Design review of the part built by this model. Coordinates are the model's own, in mm. A direction names the side the tool comes from. Give positions to 0.01 mm unless a question says otherwise; leave off trailing zeros. Write each loop counter-clockwise with the first axis right and the second up, starting at its lowest first coordinate (ties: lowest second). Pieces come first, ordered by that corner, then holes. Notation, with made-up numbers: (8, -36.5) - (50, -36.5) arc R11 ccw to (50, -30.5) - close; hole circle Ø3 at (-30.5, -18). An arc over 180 degrees is marked (long way). Write each question's results on one line, items separated by ' | '. Start each with the question number.
from build123d import *

# Parameters (mm, degrees)
SKETCH_1_W          = 10
SKETCH_1_H          = 10
SKETCH_1_W_2        = 8
SKETCH_1_H_2        = 8
EXTRUDE_1_DEPTH     = 225
SKETCH_2_R          = 2.1
CUT_EXTRUDE_1_DEPTH = 226.277606521
SKETCH_3_R          = 2.1
CUT_EXTRUDE_2_DEPTH = 226.277606521


with BuildPart() as part:
    # ｽｹｯﾁ1 → 押し出し-薄板1 (new body)
    with BuildSketch(Plane(origin=(0, 0, 0), x_dir=(0, 0, -1), z_dir=(1, 0, 0))):
        Rectangle(SKETCH_1_W, SKETCH_1_H)
        Rectangle(SKETCH_1_W_2, SKETCH_1_H_2, mode=Mode.SUBTRACT)
    extrude(amount=EXTRUDE_1_DEPTH)

    # ｽｹｯﾁ2 → ｶｯﾄ - 押し出し1 (cut, through all)
    with BuildSketch(Plane(origin=(0, 5, 0), x_dir=(1, 0, 0), z_dir=(0, 1, 0))):
        with Locations(Location((195, 0, 0), (0, 0, 270))):
            Circle(SKETCH_2_R)
        with Locations(Location((220, 0, 0), (0, 0, 270))):
            Circle(SKETCH_2_R)
        with Locations(Location((5, 0, 0), (0, 0, 270))):
            Circle(SKETCH_2_R)
        with Locations(Location((30, 0, 0), (0, 0, 270))):
            Circle(SKETCH_2_R)
    extrude(amount=-CUT_EXTRUDE_1_DEPTH, mode=Mode.SUBTRACT)

    # ｽｹｯﾁ3 → ｶｯﾄ - 押し出し2 (cut, through all)
    with BuildSketch(Plane(origin=(0, 5, 0), x_dir=(1, 0, 0), z_dir=(0, 1, 0))):
        with Locations(Location((95, 0, 0), (0, 0, 270))):
            Circle(SKETCH_3_R)
    extrude(amount=-CUT_EXTRUDE_2_DEPTH, mode=Mode.SUBTRACT)


solid = part.part
Q1. The part is to be moulded in two halves that separate along Z. For faces 1 (the face through (111, 0, 5)), 2 (the face through (0, 0.1, 4.5)), 3 (the face through (111, 0, 4)), say which applies: +Z half, -Z half, draft (parallel to the pull), parting line (faces both ways), or undercut.
Q2. Add section B-B on x = 95. State the section outline as (y, z) points, plus the area to 3 significant figures.
Q3. Insertion check: P1, Ø2.5, axis at x = 5, z = 0, coming from the +Y side. The pin has a flat end and moves straight along its axis. Give the tip position at first contact, or say it passes through.
Q4. For line 1 along X through (y, z) = (4.55, 0); line 2 along Y through (x, z) = (167.5, -3.5), list the stretches that pass through material, from the lowest coordinate up. Write a range as [from, to].
Q5. Add section C-C on x = 179. State the section outline as (y, z) points, plus the area to 3 significant figures.
Q6. Add section D-D on z = 0. Count the separate pieces of the cut face and the enclosed holes in it, plus the area to 3 significant figures.
Q7. Machinability: for faces 4 (the face through (111, 0, -4)), 5 (the face through (197.082, -4.493, -0.273)), which of the approach directions +Z, -Z, +X, -X, +Y, -Y give a long, thin tool a straight path to every point of the face, cutting with its end or side? Answer none if there is none.
Q8. Add section A-A on y = 2.5. State the section outline as (x, z) points.
Result:
1) face 1: +Z half | face 2: draft | face 3: undercut
2) outline: (-5, -5) - (5, -5) - (5, -2.1) - (4, -2.1) - (4, -4) - (-4, -4) - (-4, -2.1) - (-5, -2.1) - close; (-5, 2.1) - (-4, 2.1) - (-4, 4) - (4, 4) - (4, 2.1) - (5, 2.1) - (5, 5) - (-5, 5) - close | area: 27.6 mm²
3) P1: passes through
4) line 1: x = [0, 2.9], [7.1, 27.9], [32.1, 92.9], [97.1, 192.9], [197.1, 217.9], [222.1, 225] | line 2: y = [-5, -4], [4, 5]
5) outline: (-5, -5) - (5, -5) - (5, 5) - (-5, 5) - close; hole (-4, -4) - (4, -4) - (4, 4) - (-4, 4) - close | area: 36.0 mm²
6) separate pieces: 12 | enclosed holes: 0 | area: 408 mm²
7) face 4: +X, -X | face 5: +Y, -Y
8) outline: (0, -5) - (225, -5) - (225, -4) - (0, -4) - close; (0, 4) - (225, 4) - (225, 5) - (0, 5) - close
